from build123d import *

# Parameters (mm, degrees)
SKETCH1_R           = 12.0000014
SKETCH1_R_2         = 11.999960371
SKETCH1_R_3         = 15.875
BOSS_EXTRUDE1_DEPTH = 6.35


with BuildPart() as part:
    # Sketch1 → Boss-Extrude1 (new body)
    with BuildSketch(Plane.XY):
        with BuildLine():
            add(Edge.make_bspline(
                [(1361.096561672, 1948.863494174), (1364.400827848, 1984.023171072), (1498.613211066, 2056.462277252), (1658.30760281, 1990.654880293), (1706.236065024, 1885.549246122)],
                knots=[0, 0, 0, 0, 0.219674411, 1, 1, 1, 1], degree=3))
            ThreePointArc((1706.236065024, 1885.549246122), (1792.519416012, 1472.613494175), (1706.236065024, 1059.677742228))
            add(Edge.make_bspline(
                [(1361.096561672, 996.363494176), (1364.400827848, 961.203817278), (1498.613211066, 888.764711097), (1658.30760281, 954.572108057), (1706.236065024, 1059.677742228)],
                knots=[0, 0, 0, 0, 0.219674411, 1, 1, 1, 1], degree=3))
            Line((1361.096561672, 996.363494176), (1361.096561672, 1948.863494174))
        make_face()
        with Locations((1453.664967726, 1842.614506828)):
            Circle(SKETCH1_R, mode=Mode.SUBTRACT)
        with Locations((1480.66492898, 1776.364555337)):
            Circle(SKETCH1_R_2, mode=Mode.SUBTRACT)
        with Locations((1462.664975126, 1807.614576828)):
            Circle(SKETCH1_R, mode=Mode.SUBTRACT)
        with Locations((1528.664893926, 1776.364575828)):
            Circle(SKETCH1_R, mode=Mode.SUBTRACT)
        with Locations((1510.664904526, 1807.614576828)):
            Circle(SKETCH1_R, mode=Mode.SUBTRACT)
        with Locations((1501.664897126, 1842.614506828)):
            Circle(SKETCH1_R, mode=Mode.SUBTRACT)
        with Locations((1424.596561672, 1405.938494174)):
            Circle(SKETCH1_R_3, mode=Mode.SUBTRACT)
        with Locations((1424.596561672, 1450.388494174)):
            Circle(SKETCH1_R_3, mode=Mode.SUBTRACT)
        with Locations((1424.596561672, 1494.838494174)):
            Circle(SKETCH1_R_3, mode=Mode.SUBTRACT)
        with Locations((1424.596561672, 1539.288494174)):
            Circle(SKETCH1_R_3, mode=Mode.SUBTRACT)
        with Locations((1501.664897126, 1283.814506828)):
            Circle(SKETCH1_R, mode=Mode.SUBTRACT)
        with Locations((1480.664970258, 1217.564562981)):
            Circle(SKETCH1_R, mode=Mode.SUBTRACT)
        with Locations((1528.664901326, 1217.564562981)):
            Circle(SKETCH1_R, mode=Mode.SUBTRACT)
        with Locations((1453.664901229, 1283.814468752)):
            Circle(SKETCH1_R, mode=Mode.SUBTRACT)
        with Locations((1508.664375126, 1712.614512828)):
            Circle(SKETCH1_R, mode=Mode.SUBTRACT)
        with Locations((1508.664375126, 1153.814512828)):
            Circle(SKETCH1_R, mode=Mode.SUBTRACT)
        with Locations((1462.664908629, 1248.814538752)):
            Circle(SKETCH1_R, mode=Mode.SUBTRACT)
        with Locations((1510.664904526, 1248.814576828)):
            Circle(SKETCH1_R, mode=Mode.SUBTRACT)
    extrude(amount=BOSS_EXTRUDE1_DEPTH)


solid = part.part
The model under review builds one solid part; all positions refer to its coordinate system, in mm. Round coordinates to 2 decimals unless told otherwise and drop trailing zeros. Loops run counter-clockwise (first coordinate to the right, second up) from the corner with the lowest first, then second, coordinate; pieces in that order, holes last. Notation, with made-up numbers: (9, 68.5) -> (52, 68.5) arc R17 cw to (52, 95.5) -> close; hole circle Ø9 at (72, 87.25). An arc over 180 degrees is marked (long way). Answer as CSV lines item,"result".
1) To check wall thickness, follow line 1 along Y through (x, z) = (1452.5, 5.5); line 2 along Y through (x, z) = (1528.5, 1); line 3 along Y through (x, z) = (1529.5, 1.75). State the ranges of each line that lie inside material, in increasing order. Write a range as from..to.
Geometry results:
line 1,"y = 929.52..1242.44, 1255.19..1271.87, 1295.76..1801.24, 1813.99..1830.67, 1854.56..2015.71"
line 2,"y = 928.99..1205.57, 1229.56..1764.37, 1788.36..2016.24"
line 3,"y = 929.14..1205.59, 1229.54..1764.39, 1788.34..2016.08"
2) For P1, Ø6, axis at x = 1485.5, y = 1423, coming from the -Z side; P2, Ø1, axis at x = 1717, z = 3.5, coming from the -Y side, all flat-tipped, find the tip position at first contact; note any pin that passes through.
Geometry results:
P1,"stops at z = 0"
P2,"stops at y = 1084.01"
3) Add section C-C on y = 1600. Write out the cut boundary in (x, z), plus the area to 3 significant figures.
Geometry results:
outline,"(1361.1, 0) -> (1784.62, 0) -> (1784.62, 6.35) -> (1361.1, 6.35) -> close"
area,"2,690 mm²"
4) Add section A-A on x = 1426.5. State how many separate pieces and enclosed holes the cut face has, plus the area to 3 significant figures.
Geometry results:
separate pieces,"5"
enclosed holes,"0"
area,"6,020 mm²"
5) Add section D-D on x = 1724. Write out the cut boundary in (y, z) (3 decimals).
Geometry results:
outline,"(1102.982, 0) -> (1842.245, 0) -> (1842.245, 6.35) -> (1102.982, 6.35) -> close"
6) Draft analysis for pull direction Y (two halves, no side actions). For faces 1 (the face through (1520.11, 1157.42, 3.13)), 2 (the face through (1532, 1481, 6.35)), state which applies: pulls with the +Y half, pulls with the -Y half, needs draft (parallel to the pull), parting line crosses it, or undercut.
Geometry results:
face 1,"undercut"
face 2,"needs draft"
